Verification items for the finished model (mm, model axes). Face numbers are marked on the shaded views. A direction names the side the tool comes from. Coordinates: 2 decimals unless noted, no trailing zeros. Order: outer loops, then holes, each group sorted by start corner. A loop starts at its lowest first (then second) coordinate and runs counter-clockwise, first axis right, second up.
Q1. Cross-section at D-D, the plane y = 2. Record the boundary of the cut face in (x, z), and give its area (3 significant figures).
Q2. Depth check by flat-ended pin: P1, Ø6, axis at y = 2.5, z = 12, coming from the -X side; P2, Ø2.5, axis at x = -12.5, z = 8, coming from the +Y side; P3, Ø5, axis at y = 4.5, z = 8, coming from the -X side. Enter the tip coordinate at first touch or a pass-through.
Q3. Cross-section at B-B, the plane z = 10.75. Record the boundary of the cut face in (x, y), and give its area (3 significant figures).
Q4. Draft check along X on the marked faces 1, 2 and 3. Enter one of: pulls with the +X half, pulls with the -X half, needs draft (parallel to the pull), parting line crosses it, or undercut.
Q5. Thickness scan on line 1 (X direction, y = -2.75, z = 10.75); line 2 (Y direction, x = -11.5, z = 8); line 3 (Y direction, x = 1, z = 1). Record the ranges inside material, lowest first.
Q6. Cross-section at A-A, the plane y = -3.5. Record the boundary of the cut face in (x, z), and give its area (3 significant figures).
Q7. Cross-section at C-C, the plane x = -11. Record the boundary of the cut face in (y, z), and give its area (3 significant figures).
Q8. Set-up check for the marked faces 4, 5 and 6: record each of +Z, -Z, +X, -X, +Y, -Y from which the full face is reachable in a straight line by a thin tool's end or side.
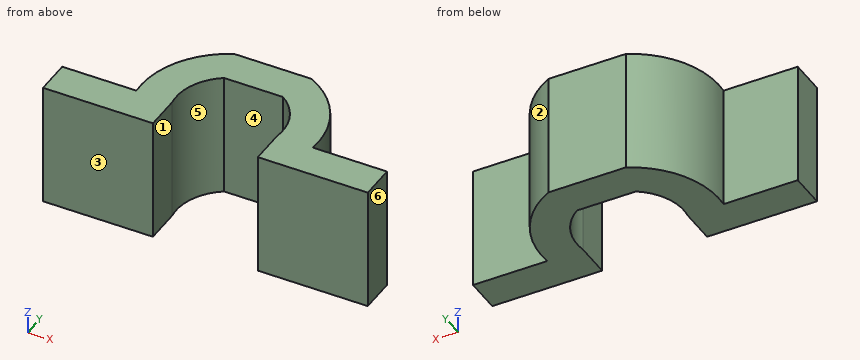
from build123d import *

# Parameters (mm, degrees)
SALIENTE_EXTRUIR2_DEPTH = 14


with BuildPart() as part:
    # Croquis1 → Saliente-Extruir2 (new body)
    with BuildSketch(Plane.XY):
        with BuildLine():
            Line((-3.31662479, 5), (3.31662479, 5))
            ThreePointArc((3.31662479, 5), (5.505516182, 2.385223588), (5.916079783, -1))
            Line((5.916079783, -1), (5.916079783, -5))
            Line((5.916079783, -5), (18.31662479, -5))
            Line((18.31662479, -5), (18.31662479, -1))
            Line((18.31662479, -1), (9.949874371, -1))
            ThreePointArc((9.949874371, -1), (8.728416147, 4.88003602), (4.358898944, 9))
            Line((4.358898944, 9), (-4.358898944, 9))
            ThreePointArc((-4.358898944, 9), (-8.728416147, 4.88003602), (-9.949874371, -1))
            Line((-9.949874371, -1), (-18.31662479, -1))
            Line((-18.31662479, -1), (-18.31662479, -5))
            Line((-18.31662479, -5), (-5.916079783, -5))
            Line((-5.916079783, -5), (-5.916079783, -1))
            ThreePointArc((-5.916079783, -1), (-5.505516182, 2.385223588), (-3.31662479, 5))
        make_face()
    extrude(amount=SALIENTE_EXTRUIR2_DEPTH)


solid = part.part
Check values:
1. outline: (-9.8, 0) - (-5.66, 0) - (-5.66, 14) - (-9.8, 14) - close; (5.66, 0) - (9.8, 0) - (9.8, 14) - (5.66, 14) - close
1. area: 116 mm2
2. P1: stops at x = -10
2. P2: stops at y = -1
2. P3: stops at x = -9.8
3. outline: (-18.32, -5) - (-5.92, -5) - (-5.92, -1) arc R6 cw to (-3.32, 5) - (3.32, 5) arc R6 cw to (5.92, -1) - (5.92, -5) - (18.32, -5) - (18.32, -1) - (9.95, -1) arc R10 ccw to (4.36, 9) - (-4.36, 9) arc R10 ccw to (-9.95, -1) - (-18.32, -1) - close
3. area: 206 mm2
4. face 1: undercut
4. face 2: pulls with the +X half
4. face 3: needs draft
5. line 1: x = -18.32 to -5.92, 5.92 to 18.32
5. line 2: y = -5 to -1
5. line 3: y = 5 to 9
6. outline: (-18.32, 0) - (-5.92, 0) - (-5.92, 14) - (-18.32, 14) - close; (5.92, 0) - (18.32, 0) - (18.32, 14) - (5.92, 14) - close
6. area: 347 mm2
7. outline: (-5, 0) - (-1, 0) - (-1, 14) - (-5, 14) - close
7. area: 56.0 mm2
8. face 4: +Z, -Z, -Y
8. face 5: +Z, -Z
8. face 6: +Z, -Z, +X, +Y, -Y
